For this review, take the finished solid that the model builds, in its own axes (mm). Face numbers are marked on the shaded views. A direction names the side the tool comes from. Give positions to 0.01 mm unless a question says otherwise; leave off trailing zeros. Write each loop counter-clockwise with the first axis right and the second up, starting at its lowest first coordinate (ties: lowest second). Pieces come first, ordered by that corner, then holes.
from build123d import *

# Parameters (mm, degrees)
DODANIE_WYCI_GNI_CIE1_DEPTH     = 17
ZAOKR_GLENIE1_R                 = 2
DODANIE_WYCI_GNI_CIE2_DEPTH     = 2
ZAOKR_GLENIE2_R                 = 1
ZAOKR_GLENIE3_R                 = 1
WYTNIJ_WYCI_GNI_CIE1_DEPTH      = 32.35628887
WYTNIJ_WYCI_GNI_CIE1_DEPTH_BACK = 32.35628887
SZKIC4_R                        = 2.1
WYTNIJ_WYCI_GNI_CIE2_DEPTH      = 31.967447566
SZKIC6_R                        = 2.1
SZKIC6_R_2                      = 1.25
DODANIE_WYCI_GNI_CIE3_DEPTH     = 0.51


with BuildPart() as part:
    # Szkic1 → Dodanie-wyciągnięcie1 (new body)
    with BuildSketch(Plane.XY):
        Polygon((1.783068787, -4.564092652), (-0.653727134, 7.430712848), (-12.25993137, 11.317788426), (-21.429339686, 3.210058505), (-18.992543765, -8.784746995), (-7.386339528, -12.671822573), align=None)
    extrude(amount=DODANIE_WYCI_GNI_CIE1_DEPTH)

    # Zaokrąglenie1
    zaokr_glenie1_edges = [part.edges().sort_by_distance(p)[0] for p in [
        (-7.386339528, -12.671822573, 8.5),
        (-18.992543765, -8.784746995, 8.5),
        (-21.429339686, 3.210058505, 8.5),
        (-12.25993137, 11.317788426, 8.5),
        (-0.653727134, 7.430712848, 8.5),
        (1.783068787, -4.564092652, 8.5),
    ]]
    fillet(zaokr_glenie1_edges, radius=ZAOKR_GLENIE1_R)

    # Szkic3 → Dodanie-wyciągnięcie2 (add)
    with BuildSketch(Plane.XY.offset(17)):
        Polygon((-0.091452095, 7.927884965), (-12.409357535, 12.053318952), (-22.141040889, 3.448416913), (-19.554818803, -9.281919113), (-7.236913363, -13.407353099), (2.494769991, -4.80245106), align=None)
    extrude(amount=-DODANIE_WYCI_GNI_CIE2_DEPTH)

    # Zaokrąglenie2
    zaokr_glenie2_edges = [part.edges().sort_by_distance(p)[0] for p in [
        (-6.456829252, 9.374250637, 0),
        (-2.80163537, -8.617957613, 0),
        (-13.189441647, -10.728284784, 0),
        (-20.210941725, -2.787344245, 0),
        (-16.844635528, 7.263923465, 0),
        (0.564670827, 1.433310098, 0),
        (-12.198333493, 11.014581025, 0),
        (-21.135955436, 3.111800131, 0),
        (-18.760757392, -8.579797968, 0),
        (-7.447937406, -12.368615173, 0),
        (1.489684537, -4.465834278, 0),
        (-0.885513507, 7.225763821, 0),
    ]]
    fillet(zaokr_glenie2_edges, radius=ZAOKR_GLENIE2_R)

    # Zaokrąglenie3
    zaokr_glenie3_edges = [part.edges().sort_by_distance(p)[0] for p in [
        (1.201658948, 1.562716953, 17),
        (-6.250404815, 9.990601959, 17),
        (-17.275199212, 7.750867932, 17),
        (-20.847929846, -2.9167511, 17),
        (-13.395866083, -11.344636106, 17),
        (-2.371071686, -9.10490208, 17),
    ]]
    fillet(zaokr_glenie3_edges, radius=ZAOKR_GLENIE3_R)

    # Szkic4 → Wytnij-wyciągnięcie1 (cut, two sides: drawn at the far end of the back side and taken through both)
    with BuildSketch(Plane(origin=(-0.257260592, 1.266331223, 0), x_dir=(0.9799817241599056, 0.19908746899937949, 0), z_dir=(-0.19908746899937946, 0.9799817241599055, 0)).offset(-WYTNIJ_WYCI_GNI_CIE1_DEPTH_BACK)):
        with Locations(Location((-9.76127883, -5.05, 0), (0, 0, 241.563109851))):
            Circle(SZKIC4_R)
    extrude(amount=WYTNIJ_WYCI_GNI_CIE1_DEPTH + WYTNIJ_WYCI_GNI_CIE1_DEPTH_BACK, mode=Mode.SUBTRACT)

    # Szkic5 → Wytnij-wyciągnięcie2 (cut, through all)
    with BuildSketch(Plane.XY.offset(17)):
        Polygon((-18.116731906, 1.847365587), (-3.172010612, 4.88344949), (-1.529538993, -3.201399735), (-16.474260286, -6.237483637), align=None)
    extrude(amount=-WYTNIJ_WYCI_GNI_CIE2_DEPTH, mode=Mode.SUBTRACT)

    # Szkic6 → Dodanie-wyciągnięcie3 (add)
    with BuildSketch(Plane(origin=(-1.078496401, 5.308755835, 0), x_dir=(0.9799817241599059, 0.19908746899937776, 0), z_dir=(0.19908746899937776, -0.9799817241599059, 0))):
        with Locations(Location((-9.76127883, 5.05, 0), (0, 0, 241.563109851))):
            Circle(SZKIC6_R)
        with Locations((-9.76127883, 5.05)):
            Circle(SZKIC6_R_2, mode=Mode.SUBTRACT)
    dodanie_wyci_gni_cie3 = extrude(amount=-DODANIE_WYCI_GNI_CIE3_DEPTH)

    # Lustro1: Dodanie-wyciągnięcie3 across plane
    add(dodanie_wyci_gni_cie3.mirror(Plane(origin=(-0.257260592, 1.266331223, 0), x_dir=(0, 0, 1), z_dir=(-0.19908746899937949, 0.9799817241599056, 0))))


solid = part.part
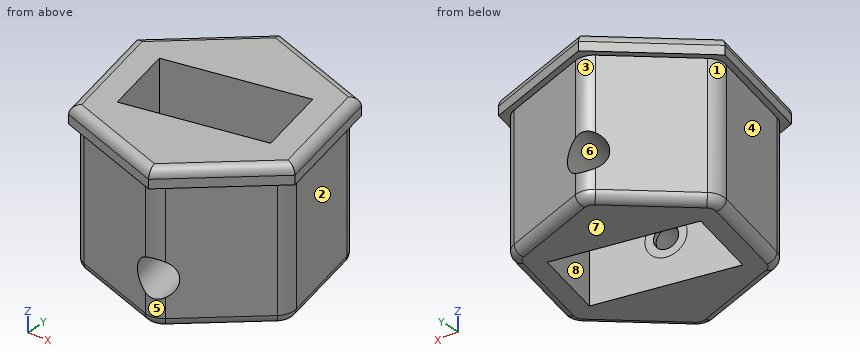
(1) The part is to be moulded in two halves that separate along X. For the marked faces 5, 6, 7 and 8, say which applies: +X half, -X half, draft (parallel to the pull), parting line (faces both ways), or undercut.
(2) Tool access review of the marked faces 1, 2, 3 and 4: name each direction out of +Z, -Z, +X, -X, +Y, -Y from which nothing blocks a thin tool from reaching the whole face with its end or side.
(3) We need section A-A (z = 9.25). Write out the cut boundary in (x, y) (1 decimal), and give its area (3 significant figures).
(4) We need section B-B (z = 4.25). Write out the cut boundary in (x, y), and give its area (3 significant figures).
(5) For L1, parallel to Z at x = -12, y = 9.5; L2, parallel to X at y = 0.25, z = 13.5; L3, parallel to X at y = -0.25, z = 12.75, list the stretches that pass through material, from the lowest coordinate up.
(6) Clearance check with flat-ended pins moving along their axes: pin 1 Ø2 at (y, z) = (8, 4.5) entering from +X; pin 2 Ø8 at (x, z) = (-7.5, 13.5) entering from +Y; pin 3 Ø10 at (x, y) = (-16.5, -4) entering from -Z; pin 4 Ø4 at (x, y) = (-1, -9) entering from -Z. State where each tip first meets the part, or that it passes through.
The answers:
1. face 5: parting line
1. face 6: undercut
1. face 7: draft
1. face 8: undercut
2. face 1: -Z, -X
2. face 2: -Z, +X, +Y
2. face 3: -Z, +Y
2. face 4: -Z, -X, -Y
3. outline: (-21.2, 2.1) - (-19.2, -7.7) arc R2 ccw to (-17.9, -9.2) - (-8.5, -12.3) arc R2 ccw to (-6.5, -11.9) - (0.9, -5.3) arc R2 ccw to (1.6, -3.4) - (-0.4, 6.3) arc R2 ccw to (-1.7, 7.8) - (-11.2, 11) arc R2 ccw to (-13.1, 10.6) - (-20.6, 4) arc R2 ccw to start; hole (-18.1, 1.8) - (-16.5, -6.2) - (-1.5, -3.2) - (-3.2, 4.9) - close
3. area: 262 mm2
4. outline: (-21.2, 2.08) - (-19.22, -7.65) arc R2 ccw to (-17.9, -9.15) - (-9.51, -11.96) - (-10.8, -5.61) - (-9.84, -5.41) - (-9.94, -4.91) - (-16.47, -6.24) - (-18.12, 1.85) - (-11.59, 3.17) - (-11.69, 3.67) - (-12.65, 3.48) - (-13.94, 9.83) - (-20.56, 3.97) arc R2 ccw to start; (-10.13, 10.61) - (-8.84, 4.25) - (-9.8, 4.06) - (-9.7, 3.56) - (-3.17, 4.88) - (-1.53, -3.2) - (-8.06, -4.53) - (-7.96, -5.03) - (-7, -4.83) - (-5.71, -11.19) - (0.92, -5.33) arc R2 ccw to (1.55, -3.43) - (-0.42, 6.3) arc R2 ccw to (-1.75, 7.8) - close
4. area: 206 mm2
5. L1: z = 0 to 2.95, 7.15 to 17
5. L2: x = -20.83 to -17.79, -2.23 to 0.81
5. L3: x = -20.73 to -17.69, -2.13 to 0.91
6. pin 1: stops at x = -0.71
6. pin 2: stops at y = 11.65
6. pin 3: stops at z = 0
6. pin 4: stops at z = 0.12
